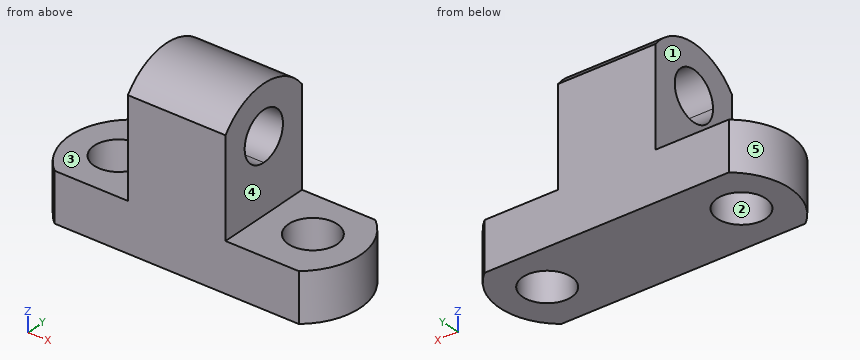
```python
from build123d import *

# Parameters (mm, degrees)
F0_W      = 76.2
F0_H      = 44.45
F1_DEPTH  = 25.4
F2_W      = 25.4
F2_H      = 31.75
F3_DEPTH  = 25.401
F5_DEPTH  = 50.801
F7_DEPTH  = 12.701
F9_DEPTH  = 12.701
F11_DEPTH = 50.501718
F13_DEPTH = 12.701
F14_R     = 6.35
F15_DEPTH = 12.701


with BuildPart() as f1:
    # F0 (on Front) → F1 (new body)
    with BuildSketch(Plane.XZ):
        with Locations((-38.1, 22.225)):
            Rectangle(F0_W, F0_H)
    extrude(amount=F1_DEPTH)

    # F2 (on face) → F3 (cut, through all)
    with BuildSketch(Plane.XZ.offset(25.4)):
        with Locations((-63.5, 28.575)):
            Rectangle(F2_W, F2_H)
        with Locations((-12.7, 28.575)):
            Rectangle(F2_W, F2_H)
    extrude(amount=-F3_DEPTH, mode=Mode.SUBTRACT)

    # F4 (on face) → F5 (cut, through all)
    with BuildSketch(Plane.YZ.offset(-25.4)):
        with BuildLine():
            Line((-25.4, 44.45), (-25.4, 38.112387))
            ThreePointArc((-25.4, 38.112387), (-12.7, 44.420951), (0, 38.112387))
            Line((0, 38.112387), (0, 44.45))
            Line((0, 44.45), (-25.4, 44.45))
        make_face()
    extrude(amount=-F5_DEPTH, mode=Mode.SUBTRACT)

    # F6 (on face) → F7 (cut, through all)
    with BuildSketch(Plane.XY.offset(12.7)):
        with BuildLine():
            Line((0, 0), (-6.35, 0))
            ThreePointArc((-6.35, 0), (-0.299282, -12.7), (-6.35, -25.4))
            Line((-6.35, -25.4), (0, -25.4))
            Line((0, -25.4), (0, 0))
        make_face()
    extrude(amount=-F7_DEPTH, mode=Mode.SUBTRACT)

    # F8 (on face) → F9 (cut, through all)
    with BuildSketch(Plane.XY.offset(12.7)):
        with BuildLine():
            Line((-76.2, -25.4), (-69.85, -25.4))
            ThreePointArc((-69.85, -25.4), (-75.870322, -12.7), (-69.85, 0))
            Line((-69.85, 0), (-76.2, 0))
            Line((-76.2, 0), (-76.2, -25.4))
        make_face()
    extrude(amount=-F9_DEPTH, mode=Mode.SUBTRACT)

    # F10 (on face) → F11 (cut, through all)
    with BuildSketch(Plane(origin=(-50.8, 0, 0), x_dir=(0, -1, 0), z_dir=(-1, 0, 0))):
        with BuildLine():
            ThreePointArc((19.05, 31.747822), (8.209872, 36.23795), (12.7, 25.397822))
            ThreePointArc((12.7, 25.397822), (17.190128, 27.257694), (19.05, 31.747822))
        make_face()
    extrude(amount=-F11_DEPTH, mode=Mode.SUBTRACT)

    # F12 (on face) → F13 (cut, through all)
    with BuildSketch(Plane.XY.offset(12.7)):
        with BuildLine():
            ThreePointArc((-56.820322, -12.7), (-63.170322, -6.35), (-69.520322, -12.7))
            ThreePointArc((-69.520322, -12.7), (-63.170322, -19.05), (-56.820322, -12.7))
        make_face()
    extrude(amount=-F13_DEPTH, mode=Mode.SUBTRACT)

    # F14 (on face) → F15 (cut, through all)
    with BuildSketch(Plane.XY.offset(12.7)):
        with Locations((-12.999282, -12.259598)):
            Circle(F14_R)
    extrude(amount=-F15_DEPTH, mode=Mode.SUBTRACT)


solid = f1.part
```
Can you work these out from the model? Positions are in its coordinate system, mm. Face numbers are marked on the shaded views. A direction names the side the tool comes from. Give positions to 0.01 mm unless a question says otherwise; leave off trailing zeros. Loops run counter-clockwise (first coordinate to the right, second up) from the corner with the lowest first, then second, coordinate; pieces in that order, holes last. Notation, with made-up numbers: M -32.5,-39.75 L 2.5,-39.75 A12 cw 2.5,-26.75 Z; hole C 82.25,-27.75 d6. An arc over 180 degrees is marked long. Use one line per item in the form item = value. Start each with the question number.
(1) On a 3-axis mill with a long thin cutter (end or side, diameter ignored), from which of +Z, -Z, +X, -X, +Y, -Y can I reach the whole of each face in a straight line? I mean the marked faces 4 and 5. Say none if no direction works.
(2) I want a section at D-D, the plane y = -4.75. Write out the boundary of the cut face in (x, z).
(3) I'm going to push flat-ended pins straight in: P1, Ø11.5, axis at y = -12.7, z = 31.75, coming from the +X side; P2, Ø2, axis at y = -9, z = 39, coming from the -X side; P3, Ø5, axis at y = -3.5, z = 12.5, coming from the -X side; P4, Ø14.5, axis at x = -13, y = -12.26, coming from the +Z side. Where does each tip first touch, or does it pass through?
(4) Please list where these lines run through material, in increasing order: line 1 (Y direction, x = -35, z = 31.5); line 2 (X direction, y = -7.25, z = 2.5); line 3 (X direction, y = -16, z = 4) (1 decimal).
(5) I want a section at A-A, the plane y = -16.25. Write out the boundary of the cut face in (x, z).
(6) I want a section at C-C, the plane z = 30. Write out the boundary of the cut face in (x, y), and give its area (3 significant figures).
(7) Thinking about a two-plate mould opening in X: for the marked faces 1, 2 and 3, which applies, released by +X, released by -X, zero draft, split by the parting line, or undercut?
(8) I want a section at B-B, the plane x = -46. Write out the boundary of the cut face in (y, z).
Worked out:
q1.face_4 = +Z, +X, +Y, -Y
q1.face_5 = +Z, -Z, -X
q2.outline = M -73.82,0 L -2.36,0 L -2.36,12.7 L -25.4,12.7 L -25.4,42.3 L -50.8,42.3 L -50.8,12.7 L -73.82,12.7 Z
q3.P1 = through
q3.P2 = -50.8
q3.P3 = -74.44
q3.P4 = 12.7
q4.line_1 = -25.4 to -19.05, -6.35 to 0
q4.line_2 = -74.94 to -66.43, -59.91 to -16.9, -9.1 to -1.23
q4.line_3 = -75.5 to -68.6, -57.7 to -18.1, -7.9 to -0.6
q5.outline = M -75.48,0 L -68.44,0 L -68.44,12.7 L -75.48,12.7 Z; M -57.91,0 L -17.94,0 L -17.94,12.7 L -25.4,12.7 L -25.4,26.48 L -50.8,26.48 L -50.8,12.7 L -57.91,12.7 Z; M -50.8,37.01 L -25.4,37.01 L -25.4,44.02 L -50.8,44.02 Z; M -8.06,0 L -0.69,0 L -0.69,12.7 L -8.06,12.7 Z
q6.outline = M -50.8,-25.4 L -25.4,-25.4 L -25.4,-18.8 L -50.8,-18.8 Z; M -50.8,-6.6 L -25.4,-6.6 L -25.4,0 L -50.8,0 Z
q6.area = 335 mm²
q7.face_1 = released by -X
q7.face_2 = undercut
q7.face_3 = zero draft
q8.outline = M -25.4,0 L 0,0 L 0,38.11 A15.94 ccw -25.4,38.11 Z; hole C -12.7,31.75 d12.7
